```python
from build123d import *

# Parameters (mm, degrees)
EXTRUDE_1_DEPTH       = 311.4
HOLE_WIZARD_10_32_1_D = 4.0386


with BuildPart() as part:
    # 草圖1 → 填料-伸長1 (new body)
    with BuildSketch(Plane(origin=(0, 0, 0), x_dir=(1, 0, 0), z_dir=(0, 1, 0))):
        with BuildLine():
            Line((-12.5, 17.5), (12.5, 17.5))
            ThreePointArc((12.5, 17.5), (30, 0), (12.5, -17.5))
            Line((12.5, -17.5), (-12.5, -17.5))
            ThreePointArc((-12.5, -17.5), (-30, 0), (-12.5, 17.5))
        make_face()
        with BuildLine():
            Line((-12.5, 15.7), (12.5, 15.7))
            ThreePointArc((12.5, 15.7), (28.2, 0), (12.5, -15.7))
            Line((12.5, -15.7), (-12.5, -15.7))
            ThreePointArc((-12.5, -15.7), (-28.2, 0), (-12.5, 15.7))
        make_face(mode=Mode.SUBTRACT)
    extrude(amount=EXTRUDE_1_DEPTH)

    # #10-32 螺紋孔1 (through all)
    with Locations(Plane.XY.offset(17.5)):
        with Locations((0, 15), (0, 30), (0, 296.4), (0, 281.4)):
            Hole(HOLE_WIZARD_10_32_1_D / 2)


solid = part.part
```
Can you work these out from the model? Positions are in its coordinate system, mm. A direction names the side the tool comes from. Coordinates: 2 decimals unless noted, no trailing zeros. Order: outer loops, then holes, each group sorted by start corner. A loop starts at its lowest first (then second) coordinate and runs counter-clockwise, first axis right, second up. Notation, with made-up numbers: (57, 82) -> (82, 82) arc R16 cw to (82, 104) -> close; hole circle Ø8 at (43.5, 0.25). An arc over 180 degrees is marked (long way). Write each question's results on one line, items separated by ' | '.
Item 1: I want a section at A-A, the plane z = 0. Write out the boundary of the cut face in (x, y), then the cut area to 3 significant figures.
Results are:
outline: (-30, 0) -> (-28.2, 0) -> (-28.2, 311.4) -> (-30, 311.4) -> close; (28.2, 0) -> (30, 0) -> (30, 311.4) -> (28.2, 311.4) -> close | area: 1,120 mm²
Item 2: If I drill on line 1 along Y through (x, z) = (0, 16.15); line 2 along X through (y, z) = (294, -0.5); line 3 along Z through (x, y) = (-7.5, 163), over which ranges is the centre line in solid material (lowest first)?
Results are:
line 1: 0 to 12.98, 17.02 to 27.98, 32.02 to 279.38, 283.42 to 294.38, 298.42 to 311.4 | line 2: -29.99 to -28.19, 28.19 to 29.99 | line 3: -17.5 to -15.7, 15.7 to 17.5
Item 3: Which directions (+Z, -Z, +X, -X, +Y, -Y) give clear straight access to the entire face, cutting with the end or side of a thin tool? Please do faces 1 (the face through (30, 154, 0)), 2 (the face through (0, 154, 15.7)).
Results are:
face 1: +X, +Y, -Y | face 2: +Y, -Y
Item 4: I want a section at C-C, the plane x = 24.5. Write out the boundary of the cut face in (y, z), then the cut area to 3 significant figures.
Results are:
outline: (0, -12.74) -> (311.4, -12.74) -> (311.4, -10.12) -> (0, -10.12) -> close; (0, 10.12) -> (311.4, 10.12) -> (311.4, 12.74) -> (0, 12.74) -> close | area: 1,630 mm²
Item 5: I'm going to push flat-ended pins straight in: pin 1 Ø12 at (x, z) = (3.5, -6.5) entering from +Y; pin 2 Ø6 at (y, z) = (144, -8) entering from +X. Where does each tip first touch, or does it pass through?
Results are:
pin 1: through | pin 2: x = 29.27
Item 6: If we mould it in two halves opening along X, with no side actions, what happens to faces 3 (the face through (0, 154, 17.5)), 4 (the face through (-28.196, 153.52, 0.345)), 5 (the face through (-30, 154, 0))? For each: +X half, -X half, draft (parallel to the pull), parting line (faces both ways), or undercut.
Results are:
face 3: draft | face 4: undercut | face 5: -X half
Item 7: I want a section at B-B, the plane y = 176.5. Write out the boundary of the cut face in (x, z), then the cut area to 3 significant figures.
Results are:
outline: (-12.5, -17.5) -> (12.5, -17.5) arc R17.5 ccw to (12.5, 17.5) -> (-12.5, 17.5) arc R17.5 ccw to start; hole (-12.5, -15.7) -> (12.5, -15.7) arc R15.7 ccw to (12.5, 15.7) -> (-12.5, 15.7) arc R15.7 ccw to start | area: 278 mm²
